```python
from build123d import *

# Parameters (mm, degrees)
SKETCH1_W          = 20
SKETCH1_H          = 60
BASE_FLANGE1_DEPTH = 1
JOG1_START         = -12.932862191
JOG1_DEPTH         = 20
JOG1_2_DEPTH       = 20


# Read off the part's stored shape, not the designer's step: Jog1
# Sheet-metal steps are written as plain solids
with BuildPart() as part:
    # Sketch1 → Base-Flange1 (new body)
    with BuildSketch(Plane(origin=(0, 0, 0), x_dir=(1, 0, 0), z_dir=(0, 1, 0))):
        with Locations((-2.932862191, 4.770318021)):
            Rectangle(SKETCH1_W, SKETCH1_H)
    extrude(amount=-BASE_FLANGE1_DEPTH)

    # Jog1 outline → Jog1 (cut)
    with BuildSketch(Plane.YZ.offset(JOG1_START)):
        with BuildLine():
            ThreePointArc((0, -4.770318021), (-0.255437354, -6.502368828), (-1, -8.086942811))
            Line((-1, -8.086942811), (-1, -34.770318021))
            Line((-1, -34.770318021), (0, -34.770318021))
            Line((0, -34.770318021), (0, -4.770318021))
        make_face()
    extrude(amount=JOG1_DEPTH, mode=Mode.SUBTRACT)

    # Jog1 2 outline → Jog1 2 (add)
    with BuildSketch(Plane.YZ.offset(JOG1_START)):
        with BuildLine():
            ThreePointArc((-1, -4.770318021), (-2.464466094, -8.305851927), (-6, -9.770318021))
            ThreePointArc((-6, -9.770318021), (-10.242640687, -11.527677334), (-12, -15.770318021))
            Line((-12, -15.770318021), (-12, -28.491558426))
            Line((-12, -28.491558426), (-11, -28.491558426))
            Line((-11, -28.491558426), (-11, -15.770318021))
            ThreePointArc((-11, -15.770318021), (-9.535533906, -12.234784115), (-6, -10.770318021))
            ThreePointArc((-6, -10.770318021), (-3.162725669, -10.057082095), (-1, -8.086942811))
            Line((-1, -8.086942811), (-1, -4.770318021))
        make_face()
    extrude(amount=JOG1_2_DEPTH)


solid = part.part
```
Work out the finished part from the listing and answer in its coordinate system (mm). A direction names the side the tool comes from. Give positions to 0.01 mm unless a question says otherwise; leave off trailing zeros. Write each loop counter-clockwise with the first axis right and the second up, starting at its lowest first coordinate (ties: lowest second). Pieces come first, ordered by that corner, then holes. Notation, with made-up numbers: (53.25, -4) -> (95.25, -4) arc R24 ccw to (95.25, 18) -> close; hole circle Ø9 at (-21, 70). An arc over 180 degrees is marked (long way). Write each question's results on one line, items separated by ' | '.
1. A tool of negligible diameter and unlimited length cuts with its end or side. For faces 1 (the flat face through (-3.1, -11.5, -28.492)), 2 (the flat face through (-3, -1, 10)), 3 (the flat face through (-3, -11, -22)), from which of +Z, -Z, +X, -X, +Y, -Y can it reach the whole face along a straight path? Write none if from no direction.
Data:
face 1: -Z, +X, -X, +Y, -Y | face 2: +Z, +X, -X, -Y | face 3: -Z, +X, -X, +Y
2. Find section B-B on z = 12.5. Determine the outline of the cut face in (x, y), and give its area (3 significant figures).
Data:
outline: (-12.93, -1) -> (7.07, -1) -> (7.07, 0) -> (-12.93, 0) -> close | area: 20.0 mm^2
3. Find section A-A on x = -11. Determine the outline of the cut face in (y, z).
Data:
outline: (-12, -28.49) -> (-11, -28.49) -> (-11, -15.77) arc R5 cw to (-6, -10.77) arc R6 ccw to (0, -4.77) -> (0, 25.23) -> (-1, 25.23) -> (-1, -4.77) arc R5 cw to (-6, -9.77) arc R6 ccw to (-12, -15.77) -> close
4. Straight lines are drawn through the part: L1, parallel to Y at x = 0, z = -21.5; L2, parallel to Y at x = 4.5, z = 11; L3, parallel to Z at x = -3.5, y = -6. For each, find the intervals that lie inside material, in ascending order.
Data:
L1: -12 to -11 | L2: -1 to 0 | L3: -10.77 to -9.77
5. Find section C-C on y = -4.25. Determine the outline of the cut face in (x, z).
Data:
outline: (-12.93, -10.51) -> (7.07, -10.51) -> (7.07, -9.45) -> (-12.93, -9.45) -> close
6. Each of these flat-tipped pins is pushed along its axis until it touches: pin 1 Ø2 at (x, z) = (-1, -17) entering from +Y; pin 2 Ø1 at (x, y) = (-1.5, -6.5) entering from -Z; pin 3 Ø4 at (x, z) = (0.5, 6) entering from -Y. Where does it stop, or does it pass through?
Data:
pin 1: y = -11 | pin 2: z = -10.87 | pin 3: y = -1
